Autodesk Inventor part; units mm, degrees
ref_plane "YZ Plane" through (0, 0, 0) normal (1, 0, 0) x (0, 1, 0)
ref_plane "XZ Plane" through (0, 0, 0) normal (0, 1, 0) x (-1, 0, 0)
ref_plane "XY Plane" through (0, 0, 0) normal (0, 0, 1) x (1, 0, 0)
sketch "Sketch1" plane through (0, 0, 0) normal (0, 0, 1) x (1, 0, 0)
  line L0 (-50.7629, 56.7485) -> (-50.7629, -66.1875)
  line L1 (-50.7629, -66.1875) -> (15.2771, -66.1875)
  line L2 (15.2771, -66.1875) -> (15.2771, 56.7485)
  line L3 (15.2771, 56.7485) -> (-50.7629, 56.7485)
  point P0 (0, 0)
  dimension "d0" = 122.936
  dimension "d1" = 66.04
extrude "Extrusion1" add sketch "Sketch1" along normal blind 35.052
sketch "Sketch2" plane through (0, 0, 35.052) normal (0, 0, 1) x (1, 0, 0)
  line L0 (-47.2069, 53.1925) -> (11.7211, 53.1925)
  line L1 (11.7211, 53.1925) -> (11.7211, -62.6315)
  line L2 (11.7211, -62.6315) -> (-47.2069, -62.6315)
  line L3 (-47.2069, -62.6315) -> (-47.2069, 53.1925)
  line L4 (15.2771, 56.7485) -> (-50.7629, 56.7485)
  line L5 (15.2771, -66.1875) -> (15.2771, 56.7485)
  line L6 (-50.7629, -66.1875) -> (15.2771, -66.1875)
  line L7 (-50.7629, 56.7485) -> (-50.7629, -66.1875)
  point P0 (0, 0)
  dimension "d4" = 3.556
  dimension "d5" = 3.556
  dimension "d6" = 3.556
  dimension "d7" = 3.556
extrude "Extrusion2" cut sketch "Sketch2" against normal blind 31.5 contours L0 L1 L2 L3
sketch "Sketch3" plane through (-50.7629, -66.1875, 0) normal (0, -1, 0) x (1, 0, 0)
  line L0 (11.556, 26.552) -> (26.556, 26.552)
  line L1 (26.556, 26.552) -> (26.556, 19.052)
  line L2 (26.556, 19.052) -> (11.556, 19.052)
  line L3 (11.556, 19.052) -> (11.556, 26.552)
  line L4 (62.484, 3.552) -> (3.556, 3.552)
  line L5 (3.556, 35.052) -> (3.556, 3.552)
  line L6 (46.484, 21.552) -> (56.484, 21.552)
  line L7 (56.484, 21.552) -> (56.484, 16.552)
  line L8 (56.484, 16.552) -> (46.484, 16.552)
  line L9 (46.484, 16.552) -> (46.484, 21.552)
  line L10 (62.484, 35.052) -> (62.484, 3.552)
  point P0 (50.7629, 0)
  dimension "d10" = 23
  dimension "d11" = 8
  dimension "d12" = 7.5
  dimension "d13" = 15
  dimension "d14" = 18
  dimension "d15" = 5
  dimension "d16" = 10
  dimension "d17" = 16
extrude "Extrusion3" cut sketch "Sketch3" against normal blind 3.56
sketch "Sketch4" plane through (0, 0, 0) normal (0, 0, -1) x (-1, 0, 0)
  line L0 (42.1269, -34.1315) -> (47.2069, -34.1315)
  line L1 (47.2069, -34.1315) -> (47.2069, -57.1315)
  line L2 (47.2069, -57.1315) -> (42.1269, -57.1315)
  line L3 (42.1269, -57.1315) -> (42.1269, -34.1315)
  line L4 (47.2069, -62.6315) -> (47.2069, 53.1925)
  line L5 (-11.7211, -62.6315) -> (47.2069, -62.6315)
  line L6 (40.2069, 30.1925) -> (47.2069, 30.1925)
  line L7 (47.2069, 30.1925) -> (47.2069, 23.1925)
  line L8 (47.2069, 23.1925) -> (40.2069, 23.1925)
  line L9 (40.2069, 23.1925) -> (40.2069, 30.1925)
  line L10 (47.2069, 53.1925) -> (-11.7211, 53.1925)
  line L11 (4.2789, 53.1925) -> (12.7789, 53.1925)
  line L12 (12.7789, 53.1925) -> (12.7789, 44.1925)
  line L13 (12.7789, 44.1925) -> (4.2789, 44.1925)
  line L14 (4.2789, 44.1925) -> (4.2789, 53.1925)
  line L15 (-11.7211, 53.1925) -> (-11.7211, -62.6315)
  point P0 (0, 0)
  dimension "d20" = 0
  dimension "d21" = 5.5
  dimension "d22" = 23
  dimension "d23" = 5.08
  dimension "d24" = 30
  dimension "d25" = 7
  dimension "d26" = 7
  dimension "d27" = 0
  dimension "d28" = 9
  dimension "d29" = 8.5
  dimension "d30" = 0
  dimension "d31" = 16
extrude "Extrusion4" cut sketch "Sketch4" against normal blind 3.56 contours L0 L1 L2 L3 | L8 L9 L6 L4 | L12 L13 L14 L10
sketch "Sketch5" plane through (-50.7629, 56.7485, 0) normal (0, 1, 0) x (1, 0, 0)
  line L0 (62.484, -14.552) -> (55.484, -14.552)
  line L1 (55.484, -14.552) -> (55.484, -3.552)
  line L2 (55.484, -3.552) -> (62.484, -3.552)
  line L3 (62.484, -3.552) -> (62.484, -14.552)
  line L4 (62.484, -35.052) -> (62.484, -3.552)
  line L5 (46.484, -3.552) -> (62.484, -3.552)
  line L6 (46.484, -4.552) -> (37.984, -4.552)
  line L7 (37.984, -4.552) -> (37.984, 2.448)
  line L8 (37.984, 2.448) -> (46.484, 2.448)
  line L9 (46.484, 2.448) -> (46.484, -4.552)
  line L10 (46.484, -3.552) -> (37.984, -3.552)
  point P0 (50.7629, 0)
  dimension "d34" = 11
  dimension "d35" = 0
  dimension "d37" = 7
  dimension "d39" = 16
  dimension "d40" = 7
  dimension "d41" = 8.5
  dimension "d50" = 1
extrude "Extrusion5" cut sketch "Sketch5" against normal blind 3.56
sketch "Sketch6" plane through (-50.7629, -66.1875, 0) normal (-1, 0, 0) x (0, 0, 1)
  line L0 (13.552, 98.38) -> (18.552, 98.38)
  line L1 (18.552, 98.38) -> (18.552, 87.38)
  line L2 (18.552, 87.38) -> (13.552, 87.38)
  line L3 (13.552, 87.38) -> (13.552, 98.38)
  line L4 (3.552, 122.936) -> (3.552, 3.556)
  line L5 (35.052, 119.38) -> (3.552, 119.38)
  point P0 (0, 66.1875)
  dimension "d44" = 15
  dimension "d45" = 5
  dimension "d46" = 11
  dimension "d47" = 32
extrude "Extrusion6" cut sketch "Sketch6" against normal blind 3.56
fillet "Fillet1" radius 1 4 edges at (15.2771, 56.7485, 17.526) (-50.7629, 56.7485, 17.526) (-50.7629, -66.1875, 17.526) (15.2771, -66.1875, 17.526)
properties part number "Smart Lock Box Bottom Correct"
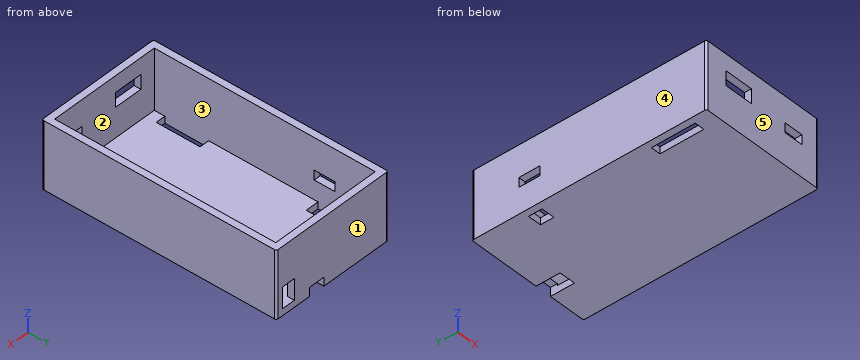
Can you work these out from the model? Positions are in its coordinate system, mm. Face numbers are marked on the shaded views. A direction names the side the tool comes from. Give positions to 0.01 mm unless a question says otherwise; leave off trailing zeros. Loops run counter-clockwise (first coordinate to the right, second up) from the corner with the lowest first, then second, coordinate; pieces in that order, holes last. Notation, with made-up numbers: (64.5, 38.25) - (88.5, 38.25) arc R24 ccw to (88.5, 68.25) - close; hole circle Ø3 at (-5.5, 39.25). An arc over 180 degrees is marked (long way). Answer as a JSON object with one key per item and string values.
Q1. Imagine slicing it at D-D on x = -20.5. Write out the boundary of the cut face in (y, z).
Geometry says:
{"outline": "(-66.19, 0) - (56.75, 0) - (56.75, 35.05) - (53.19, 35.05) - (53.19, 3.55) - (-62.63, 3.55) - (-62.63, 35.05) - (-66.19, 35.05) - close"}
Q2. Imagine slicing it at C-C on y = 16.5. Write out the boundary of the cut face in (x, z).
Geometry says:
{"outline": "(-50.76, 0) - (15.28, 0) - (15.28, 35.05) - (11.72, 35.05) - (11.72, 3.55) - (-47.21, 3.55) - (-47.21, 35.05) - (-50.76, 35.05) - close"}
Q3. Will this pin go through, and if not, where does the flat tip stop? P1, Ø3, axis at x = -9, y = 54, coming from the -Z side.
Geometry says:
{"P1": "z = 4.55"}
Q4. Which directions (+Z, -Z, +X, -X, +Y, -Y) give clear straight access to the entire face, cutting with the end or side of a thin tool? Please do the marked faces 1 and 2.
Geometry says:
{"face 1": "+Z, -Z, +X, -X, +Y", "face 2": "+Z"}
Q5. Imagine slicing it at B-B on x = -33.5. Write out the boundary of the cut face in (y, z), plus the area to 3 significant figures.
Geometry says:
{"outline": "(-66.19, 0) - (56.75, 0) - (56.75, 35.05) - (53.19, 35.05) - (53.19, 3.55) - (-62.63, 3.55) - (-62.63, 19.05) - (-66.19, 19.05) - close; (-66.19, 26.55) - (-62.63, 26.55) - (-62.63, 35.05) - (-66.19, 35.05) - close", "area": "634 mm²"}
Q6. Imagine slicing it at A-A on y = -39. Write out the boundary of the cut face in (x, z).
Geometry says:
{"outline": "(-50.76, 0) - (-47.21, 0) - (-47.21, 35.05) - (-50.76, 35.05) - close; (-42.13, 0) - (15.28, 0) - (15.28, 35.05) - (11.72, 35.05) - (11.72, 3.55) - (-42.13, 3.55) - close"}
Q7. If I drill on L1, parallel to X at y = 40, z = 12.5; L2, parallel to Y at x = -45, z = 14; L3, parallel to Z at x = -35, y = -11.5, over which ranges is the centre line in solid material (lowest first)?
Geometry says:
{"L1": "-50.76 to -47.21, 11.72 to 15.28", "L2": "-66.19 to -62.63, 53.19 to 56.75", "L3": "0 to 3.55"}
Q8. If we mould it in two halves opening along X, with no side actions, what happens to the marked faces 3, 4 and 5? For each: pulls with the +X half, pulls with the -X half, needs draft (parallel to the pull), parting line crosses it, or undercut.
Geometry says:
{"face 3": "undercut", "face 4": "pulls with the -X half", "face 5": "needs draft"}
